Design review of the part shown in the three views and the two pictorial views. Dimensions are in mm from the part's minimum x, y and z. A direction names the side the tool comes from. Round coordinates to 2 decimals unless told otherwise and drop trailing zeros. Order: outer loops, then holes, each group sorted by start corner. A loop starts at its lowest first (then second) coordinate and runs counter-clockwise, first axis right, second up. Notation, with made-up numbers: (25, 33) - (54, 33) arc R22 ccw to (54, 69) - close; hole circle Ø2 at (33, -15.5). An arc over 180 degrees is marked (long way). One line per item, written item: value.
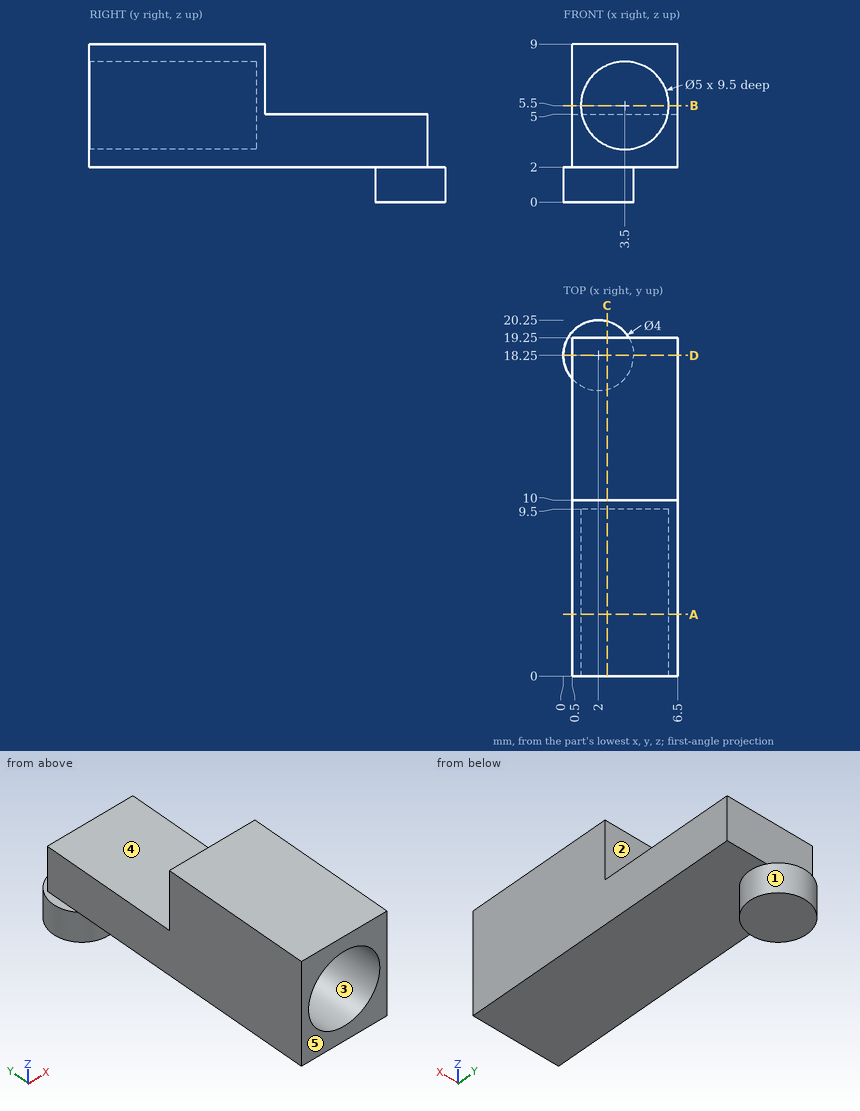
Item 1: Take a section at A-A (y = 3.5). Write out the cut boundary in (x, z), plus the area to 3 significant figures.
Returned:
outline: (0.5, 2) - (6.5, 2) - (6.5, 9) - (0.5, 9) - close; hole circle Ø5 at (3.5, 5.5)
area: 22.4 mm^2
Item 2: Take a section at D-D (y = 18.25). Write out the cut boundary in (x, z), plus the area to 3 significant figures.
Returned:
outline: (0, 0) - (4, 0) - (4, 2) - (6.5, 2) - (6.5, 5) - (0.5, 5) - (0.5, 2) - (0, 2) - close
area: 26.0 mm^2
Item 3: Machinability: for the marked faces 4 and 5, which of the approach directions +Z, -Z, +X, -X, +Y, -Y give a long, thin tool a straight path to every point of the face, cutting with its end or side? Answer none if there is none.
Returned:
face 4: +Z, +X, -X, +Y
face 5: +Z, -Z, +X, -X, -Y
Item 4: For P1, Ø2.5, axis at x = 4, z = 5, coming from the -Y side; P2, Ø2, axis at y = 9, z = 5, coming from the -X side; P3, Ø2.5, axis at x = 1.5, y = 19, coming from the +Z side, all flat-tipped, find the tip position at first contact; note any pin that passes through.
Returned:
P1: y = 9.5
P2: x = 0.5
P3: z = 5
Item 5: Take a section at C-C (x = 2.5). Write out the cut boundary in (y, z).
Returned:
outline: (0, 2) - (16.31, 2) - (16.31, 0) - (20.19, 0) - (20.19, 2) - (19.25, 2) - (19.25, 5) - (10, 5) - (10, 9) - (0, 9) - (0, 7.79) - (9.5, 7.79) - (9.5, 3.21) - (0, 3.21) - close
Item 6: Take a section at B-B (z = 5.5). Write out the cut boundary in (x, y).
Returned:
outline: (0.5, 0) - (1, 0) - (1, 9.5) - (6, 9.5) - (6, 0) - (6.5, 0) - (6.5, 10) - (0.5, 10) - close
Item 7: Wall thickness on line 1 (Z direction, x = 3.5, y = 7.25); line 2 (Z direction, x = 3.75, y = 10.75); line 3 (Y direction, x = 1.5, z = 5.75): over which ranges is each line inside the solid? List them lowest first.
Returned:
line 1: 2 to 3, 8 to 9
line 2: 2 to 5
line 3: 9.5 to 10
Item 8: The part is to be moulded in two halves that separate along X. For the marked faces 1, 2 and 3, say which applies: +X half, -X half, draft (parallel to the pull), parting line (faces both ways), or undercut.
Returned:
face 1: parting line
face 2: draft
face 3: undercut
